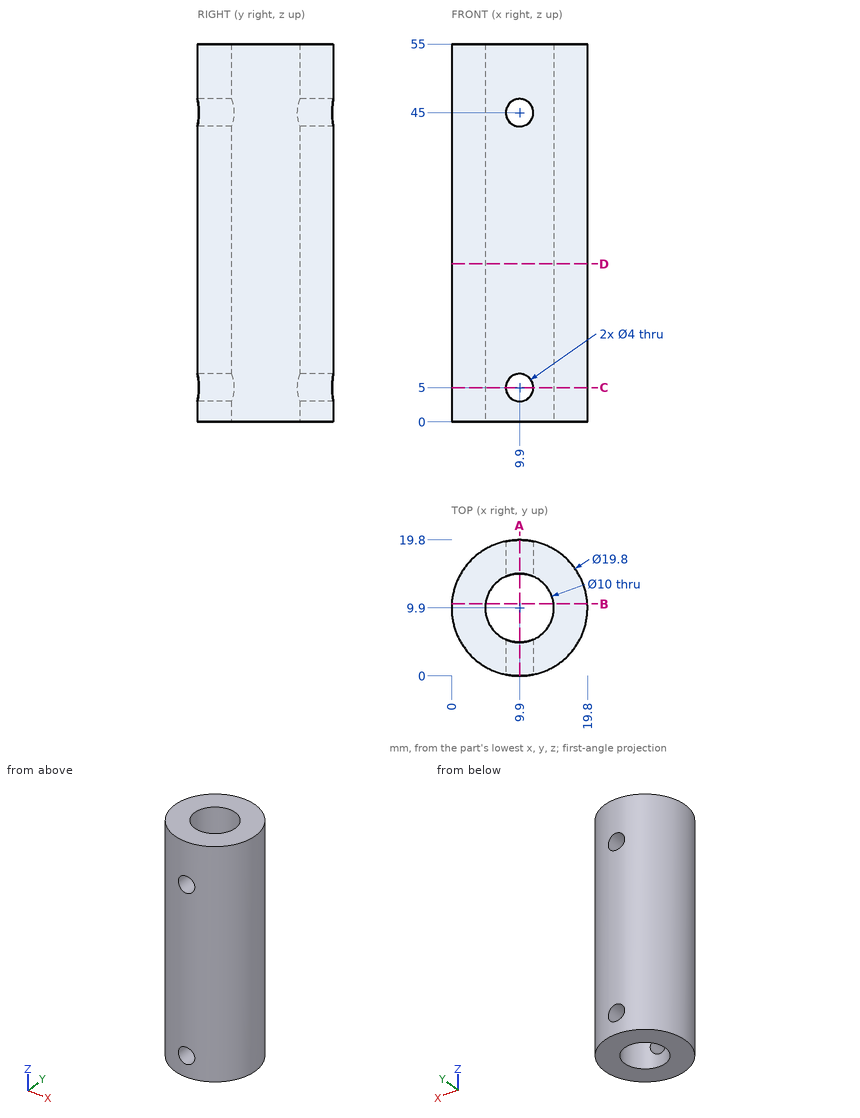
Here's the drawing with two shaded views (mm, measured from the low corner). I have some questions. Coordinates: 2 decimals unless noted, no trailing zeros. Order: outer loops, then holes, each group sorted by start corner. A loop starts at its lowest first (then second) coordinate and runs counter-clockwise, first axis right, second up.
Item 1: I need wall thicknesses on line 1 (Y direction, x = 9.9, z = 24.5); line 2 (X direction, y = 3, z = 4.5); line 3 (X direction, y = 14.5, z = 14.5). Which ranges of each line are inside material? Lowest first, please.
Result sheet:
line 1: y = 0 to 4.9, 14.9 to 19.8
line 2: x = 2.8 to 7.96, 11.84 to 17
line 3: x = 1.13 to 7.94, 11.86 to 18.67
Item 2: If we section it at C-C on z = 5: List the corners of the cut face in (x, y) for me, plus the area to 3 significant figures.
Result sheet:
outline: (7.9, 0.2) - (7.9, 5.32) arc R5 cw to (7.9, 14.48) - (7.9, 19.6) arc R9.9 ccw to start; (11.9, 0.2) arc R9.9 ccw to (11.9, 19.6) - (11.9, 14.48) arc R5 cw to (11.9, 5.32) - close
area: 190 mm2
Item 3: If we section it at A-A on x = 9.9: List the corners of the cut face in (y, z) for me, plus the area to 3 significant figures.
Result sheet:
outline: (0, 0) - (4.9, 0) - (4.9, 3) - (0, 3) - close; (0, 7) - (4.9, 7) - (4.9, 43) - (0, 43) - close; (0, 47) - (4.9, 47) - (4.9, 55) - (0, 55) - close; (14.9, 0) - (19.8, 0) - (19.8, 3) - (14.9, 3) - close; (14.9, 7) - (19.8, 7) - (19.8, 43) - (14.9, 43) - close; (14.9, 47) - (19.8, 47) - (19.8, 55) - (14.9, 55) - close
area: 461 mm2
Item 4: For P1, Ø2, axis at x = 7.5, y = 12.5, coming from the +Z side; P2, Ø2, axis at y = 12.5, z = 44.5, coming from the +X side; P3, Ø1, axis at x = 13, z = 29, coming from the -Y side; P4, Ø6, axis at y = 5, z = 48.5, coming from the +X side, each with a flat end and sliding along its axis, tell me the tip position at first contact or that it passes through.
Result sheet:
P1: passes through
P2: stops at x = 19.67
P3: stops at y = 0.35
P4: stops at x = 19.62
Item 5: If we section it at D-D on z = 23: List the corners of the cut face in (x, y) for me, plus the area to 3 significant figures.
Result sheet:
outline: circle Ø19.8 at (9.9, 9.9); hole circle Ø10 at (9.9, 9.9)
area: 229 mm2
Item 6: If we section it at B-B on y = 10.5: List the corners of the cut face in (x, z) for me, plus the area to 3 significant figures.
Result sheet:
outline: (0.02, 0) - (4.94, 0) - (4.94, 55) - (0.02, 55) - close; (14.86, 0) - (19.78, 0) - (19.78, 55) - (14.86, 55) - close
area: 541 mm2
